Can you work these out from the model? Positions are in its coordinate system, mm. A direction names the side the tool comes from. Coordinates: 2 decimals unless noted, no trailing zeros. Loops run counter-clockwise (first coordinate to the right, second up) from the corner with the lowest first, then second, coordinate; pieces in that order, holes last.
Autodesk Inventor part; units mm, degrees
ref_plane "YZ Plane" through (0, 0, 0) normal (1, 0, 0) x (0, 1, 0)
ref_plane "XZ Plane" through (0, 0, 0) normal (0, 1, 0) x (-1, 0, 0)
ref_plane "XY Plane" through (0, 0, 0) normal (0, 0, 1) x (1, 0, 0)
sketch "Sketch1" plane through (0, 0, 0) normal (0, 1, 0) x (-1, 0, 0)
  line L0 (0, 0) -> (10, 0)
  line L1 (0, 10) -> (0, 0)
  line L2 (10, 10) -> (0, 10)
  line L3 (10, 0) -> (10, 10)
  line L4 (0, 10) -> (0.05, 10)
  line L5 (0.05, 10) -> (0.05, 9.95)
  line L6 (0.05, 9.95) -> (0, 9.95)
  line L7 (0, 9.95) -> (0, 10)
  line L8 (10, 0) -> (9.95, 0)
  line L9 (9.95, 0) -> (9.95, 0.05)
  line L10 (9.95, 0.05) -> (10, 0.05)
  line L11 (10, 0.05) -> (10, 0)
  line L12 (0.05, 9.95) -> (9.95, 9.95)
  line L13 (9.95, 9.95) -> (9.95, 0.05)
  line L14 (9.95, 0.05) -> (0.05, 0.05)
  line L15 (0.05, 0.05) -> (0.05, 9.95)
  point P0 (0, 0)
  dimension "d0" = 0.05
  dimension "d1" = 0.05
  dimension "d2" = 0.05
  dimension "d3" = 0.05
extrude "Extrusion1" add sketch "Sketch1" along normal blind 5 contours L14 L15 L12 L13
sketch "Sketch2" plane through (0, 0, 0) normal (0, -1, 0) x (1, 0, 0)
  line L0 (-0.05, 0.05) -> (-9.95, 0.05)
  line L1 (-0.05, 9.95) -> (-0.05, 0.05)
  line L2 (-9.95, 9.95) -> (-0.05, 9.95)
  line L3 (-9.95, 0.05) -> (-9.95, 9.95)
  line L4 (-0.05, 5) -> (-9.95, 5)
  circle A0 centre (-5, 5) radius 7.0004
  point P0 (0, 0)
extrude "Extrusion2" add sketch "Sketch2" along normal blind 85
sketch "Sketch4" plane through (-5, -85, 5) normal (0, -1, 0) x (1, 0, 0)
  circle A0 centre (0, 0) radius 7.0004
  circle A1 centre (0, 0) radius 7.0004
  line L0 (0, -7.0004) -> (0, -12)
  line L1 (-2.5, -9.5) -> (2.5, -9.5)
  line L2 (2.5, -9.5) -> (2.5, -14.5)
  line L3 (2.5, -14.5) -> (-2.5, -14.5)
  line L4 (-2.5, -14.5) -> (-2.5, -9.5)
  line L5 (-2.5, -9.5) -> (2.5, -14.5) construction
  line L6 (2.5, -9.5) -> (-2.5, -14.5) construction
  line L7 (-7.0004, 0.0004) -> (-12.0004, 0.0004)
  line L8 (-9.5004, 2.5004) -> (-14.5004, 2.5004)
  line L9 (-14.5004, 2.5004) -> (-14.5004, -2.4996)
  line L10 (-14.5004, -2.4996) -> (-9.5004, -2.4996)
  line L11 (-9.5004, -2.4996) -> (-9.5004, 2.5004)
  line L12 (-9.5004, 2.5004) -> (-14.5004, -2.4996) construction
  line L13 (-14.5004, 2.5004) -> (-9.5004, -2.4996) construction
  line L14 (-9.5004, -2.4996) -> (-9.5004, -4.9996)
  line L15 (-14.5004, 2.5004) -> (-2.2357, 6.6338)
  line L16 (-14.5004, -2.4996) -> (-2.236, -6.6336)
  line L17 (-2.5, -14.5) -> (-6.6337, -2.2359)
  line L18 (2.5, -14.5) -> (6.6337, -2.2359)
  point P0 (5, -5)
  point P1 (-12.0004, 0.0004)
  point P2 (6.6337, -2.2359)
  point P3 (-2.2357, 6.6338)
  point P4 (-5.5251, -5.525)
  dimension "d16" = 5
  dimension "d17" = 5
  dimension "d18" = 5
  dimension "d19" = 5
  dimension "d20" = 5
  dimension "d21" = 2.5
extrude "Extrusion4" add sketch "Sketch4" against normal blind 10 contours A0 L7 L11 L8 L15 | L18 L2 L1 L0 A0 | A0 L17 L16 L14 L11 L7 | L8 L11 L10 L9 | L0 L1 L4 L17 L16 A0 | L3 L4 L1 L2 | A0 L16 L17 | L10 L14 L16
sketch "Sketch6" plane through (0, -85, 0) normal (0, -1, 0) x (1, 0, 0)
  arc A0 (1.6337, 2.7641) -> (-7.2357, 11.6338) centre (-5, 5) ccw
  line L0 (-7.2357, 11.6338) -> (-19.5004, 7.5004)
  line L1 (-19.5004, 7.5004) -> (-19.5004, 2.5004)
  line L2 (-19.5004, 2.5004) -> (-10.5251, -0.525)
  line L3 (-10.5251, -0.525) -> (-7.5, -9.5)
  line L4 (-7.5, -9.5) -> (-2.5, -9.5)
  line L5 (-2.5, -9.5) -> (1.6337, 2.7641)
  line L6 (-3, -6.5) -> (-7, -6.5)
  line L7 (-7, -6.5) -> (-7, -2.5)
  line L8 (-7, -2.5) -> (-3, -2.5)
  line L9 (-3, -2.5) -> (-3, -6.5)
  line L10 (-3, -6.5) -> (-7, -2.5) construction
  line L11 (-7, -6.5) -> (-3, -2.5) construction
  line L12 (-4, -9.5) -> (-6, -9.5)
  line L13 (-6, -9.5) -> (-6, -6.5)
  line L14 (-6, -6.5) -> (-4, -6.5)
  line L15 (-4, -6.5) -> (-4, -9.5)
  line L16 (-4, -9.5) -> (-6, -6.5) construction
  line L17 (-6, -9.5) -> (-4, -6.5) construction
  line L18 (-10.5251, -0.525) -> (-0.05, 9.95)
  line L19 (-10.5251, -0.525) -> (4.2889, -0.525) construction
  line L20 (-16.5004, 6.0004) -> (-19.5004, 6.0004)
  line L21 (-19.5004, 6.0004) -> (-19.5004, 4.0004)
  line L22 (-19.5004, 4.0004) -> (-16.5004, 4.0004)
  line L23 (-16.5004, 4.0004) -> (-16.5004, 6.0004)
  line L24 (-16.5004, 6.0004) -> (-19.5004, 4.0004) construction
  line L25 (-19.5004, 6.0004) -> (-16.5004, 4.0004) construction
  line L26 (-12.5004, 7.0004) -> (-16.5004, 7.0004)
  line L27 (-16.5004, 7.0004) -> (-16.5004, 3.0004)
  line L28 (-16.5004, 3.0004) -> (-12.5004, 3.0004)
  line L29 (-12.5004, 3.0004) -> (-12.5004, 7.0004)
  line L30 (-12.5004, 7.0004) -> (-16.5004, 3.0004) construction
  line L31 (-16.5004, 7.0004) -> (-12.5004, 3.0004) construction
  point P0 (0, 0)
  point P1 (-5, -8)
  dimension "d27" = 4
  dimension "d28" = 4
  dimension "d29" = 45
  dimension "d31" = 3
  dimension "d32" = 2
  dimension "d34" = 4
  dimension "d35" = 4
extrude "Extrusion6" cut sketch "Sketch6" against normal blind 85 contours L4 L13 L6 L15 | L6 L7 L8 L9 | L20 L23 L22 L1 | L27 L26 L29 L28 L23
properties part number "LegV2"
Item 1: I'm going to push flat-ended pins straight in: P1, Ø0.9, axis at x = -18.5, y = -82, coming from the -Z side; P2, Ø0.9, axis at y = -81.5, z = -8.5, coming from the +X side; P3, Ø5, axis at y = -8.5, z = 2, coming from the -X side. Where does each tip first touch, or does it pass through?
Results are:
P1: stops at z = 2.01
P2: stops at x = -2.01
P3: stops at x = -11.98
Item 2: Suppose I cut it at B-B, the plane x = -14.25. Please give me the cut outline in (y, z).
Results are:
outline: (-85, 0.73) - (-75, 0.73) - (-75, 3) - (-85, 3) - close; (-85, 7) - (-75, 7) - (-75, 9.27) - (-85, 9.27) - close
Item 3: We'd pull the mould along X, two halves only. Please class faces 1 (the face through (-6, -80, -8)), 2 (the face through (-18, -80, 4)), 3 (the face through (-15.08, -80.07, 1.01)), 4 (the face through (-1.77, -41.9, 11.21)): +X half, -X half, draft (parallel to the pull), parting line (faces both ways), or undercut.
Results are:
face 1: undercut
face 2: draft
face 3: -X half
face 4: parting line
Item 4: Suppose I cut it at D-D, the plane y = -61.5. Please give me the cut outline in (x, z), plus the area to 3 significant figures.
Results are:
outline: circle Ø14 at (-5, 5)
area: 154 mm2
Item 5: On a 3-axis mill with a long thin cutter (end or side, diameter ignored), from which of +Z, -Z, +X, -X, +Y, -Y can I reach the whole of each face in a straight line? I mean faces 5 (the face through (-4, -80, -8)), 6 (the face through (-5, 2, 9.95)), 7 (the face through (-12.5, -80, 5)), 8 (the face through (-11, 0, 5)). Say none if no direction works.
Results are:
face 5: -Z, +Y, -Y
face 6: +Z, +X, -X, +Y
face 7: +Y, -Y
face 8: +Z, -Z, -X, +Y
Item 6: Suppose I cut it at C-C, the plane x = -5. Please give me the cut outline in (y, z), plus the area to 3 significant figures.
Results are:
outline: (-85, -2.5) - (-75, -2.5) - (-75, -2) - (0, -2) - (0, 0.05) - (5, 0.05) - (5, 9.95) - (0, 9.95) - (0, 12) - (-85, 12) - close
area: 1,240 mm2
Item 7: I need wall thicknesses on line 1 along Y through (x, z) = (-10, 5.5); line 2 along Z through (x, y) = (-5, -18); line 3 along X through (y, z) = (-14, 5). Which ranges of each line are inside material? Lowest first, please.
Results are:
line 1: y = -85 to 0
line 2: z = -2 to 12
line 3: x = -12 to 2
Item 8: Suppose I cut it at A-A, the plane z = 5. Please give me the cut outline in (x, y).
Results are:
outline: (-12.5, -85) - (2, -85) - (2, 0) - (-0.05, 0) - (-0.05, 5) - (-9.95, 5) - (-9.95, 0) - (-12, 0) - (-12, -75) - (-12.5, -75) - close
